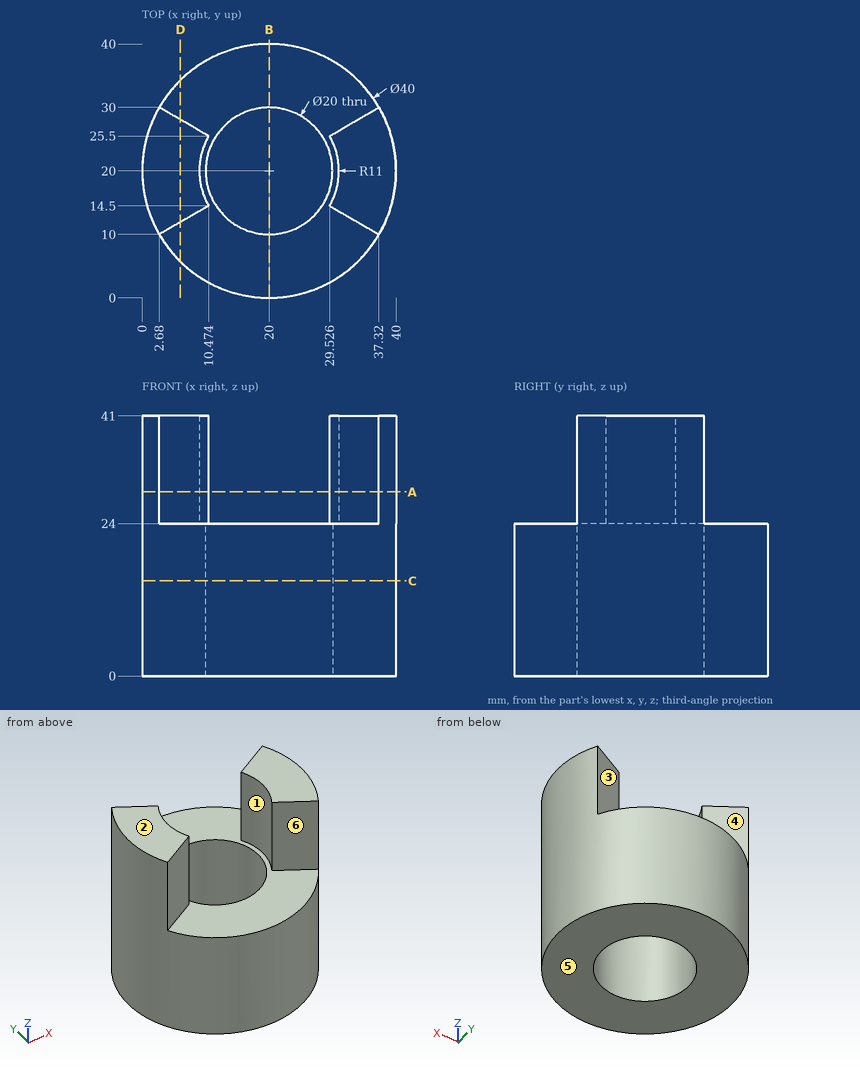
Geometry check sheet. Reference: drawing and pictorial views, mm from the part's lowest x, y, z. A direction names the side the tool comes from. Give positions to 0.01 mm unless a question says otherwise; leave off trailing zeros. Write each loop counter-clockwise with the first axis right and the second up, starting at its lowest first coordinate (ties: lowest second). Pieces come first, ordered by that corner, then holes. Notation, with made-up numbers: (82, 15) - (111, 15) arc R21 cw to (111, 27) - close; hole circle Ø1 at (-4, 22). An arc over 180 degrees is marked (long way). Put each result on its own line as item: value.
Q1. Section check A-A on z = 29. Record the cut outline in (x, y).
Result:
outline: (2.68, 10) - (10.47, 14.5) arc R11 cw to (10.47, 25.5) - (2.68, 30) arc R20 ccw to start; (29.53, 14.5) - (37.32, 10) arc R20 ccw to (37.32, 30) - (29.53, 25.5) arc R11 cw to start
Q2. Set-up check for the marked faces 4, 5 and 6: record each of +Z, -Z, +X, -X, +Y, -Y from which the full face is reachable in a straight line by a thin tool's end or side.
Result:
face 4: +Z, +Y
face 5: -Z, +X, -X, +Y, -Y
face 6: +Z, -Y
Q3. Section check C-C on z = 15. Record the cut outline in (x, y).
Result:
outline: circle Ø40 at (20, 20); hole circle Ø20 at (20, 20)
Q4. Section check B-B on x = 20. Record the cut outline in (y, z).
Result:
outline: (0, 0) - (10, 0) - (10, 24) - (0, 24) - close; (30, 0) - (40, 0) - (40, 24) - (30, 24) - close
Q5. Mould release check, pull along Y, two halves, no side actions. Record for the marked faces 1, 2 and 3: released by +Y, released by -Y, zero draft, split by the parting line, or undercut.
Result:
face 1: undercut
face 2: zero draft
face 3: released by +Y
Q6. Scan lines: probe 1 along Y at (x, z) = (20, 16.5); probe 2 along X at (y, z) = (19.5, 11.5); probe 3 along Z at (x, y) = (25, 8). Record each from-to range of solid material in increasing order. Write a range as from..to.
Result:
probe 1: 0..10, 30..40
probe 2: 0.01..10.01, 29.99..39.99
probe 3: 0..24
Q7. Section check D-D on x = 6. Record the cut outline in (y, z).
Result:
outline: (5.72, 0) - (34.28, 0) - (34.28, 24) - (28.08, 24) - (28.08, 41) - (11.92, 41) - (11.92, 24) - (5.72, 24) - close
Q8. Depth check by flat-ended pin: P1, Ø10, axis at x = 23, y = 9, coming from the -Z side; P2, Ø2, axis at x = 13, z = 23, coming from the +Y side; P3, Ø4, axis at x = 33, z = 30.5, coming from the +Y side; P4, Ø1.5, axis at y = 26.5, z = 17, coming from the -X side (1 decimal). Enter the tip coordinate at first touch or a pass-through.
Result:
P1: z = 0
P2: y = 39.08
P3: y = 28.66
P4: x = 0.8
